Can you work these out from the model? Positions are in its coordinate system, mm. A direction names the side the tool comes from. Give positions to 0.01 mm unless a question says otherwise; leave off trailing zeros. Write each loop counter-clockwise with the first axis right and the second up, starting at its lowest first coordinate (ties: lowest second). Pieces come first, ordered by that corner, then holes.
```python
from build123d import *
from build123d.topology import SkipClean

# Parameters (mm, degrees)
BOSS_EXTRUDE1_DEPTH       = 25.4
F_8_0_18_DIAMETER_HOLE1_D = 4.572
SKETCH8_W                 = 22.225
SKETCH8_H                 = 53.34
CUT_EXTRUDE1_DEPTH        = 74.933200255
CUT_EXTRUDE2_DEPTH        = 74.933200255
FILLET1_R                 = 3.175
FILLET3_R                 = 0.508
FILLET4_R                 = 6.35


with BuildPart() as part:
    # Sketch1 → Boss-Extrude1 (new body)
    with BuildSketch(Plane(origin=(0, 0, 0), x_dir=(0, 0, -1), z_dir=(1, 0, 0))):
        with BuildLine():
            Line((0, 0), (0, 53.34))
            Line((0, 53.34), (-22.225, 53.34))
            Line((-22.225, 53.34), (-22.225, 46.482))
            ThreePointArc((-22.225, 46.482), (-2.413, 26.67), (-22.225, 6.858))
            Line((-22.225, 6.858), (-22.225, 0))
            Line((-22.225, 0), (0, 0))
        make_face()
    boss_extrude1 = extrude(amount=BOSS_EXTRUDE1_DEPTH)

    # #8 (0.18) Diameter Hole1 (through all)
    with Locations(Plane.XY.offset(22.225)):
        with Locations((4.7625, 49.911), (20.6375, 49.911), (20.6375, 3.429), (4.7625, 3.429)):
            f_8_0_18_diameter_hole1 = Hole(F_8_0_18_DIAMETER_HOLE1_D / 2)

    # Mirror1: Boss-Extrude1, #8 (0.18) Diameter Hole1 across plane
    with SkipClean():  # the faces are left unmerged after this step: merging them gives an invalid solid
        add(boss_extrude1.mirror(Plane(origin=(25.4, 53.34, 22.225), x_dir=(1, 0, 0), z_dir=(0, 0, -1))))
        add(f_8_0_18_diameter_hole1.mirror(Plane(origin=(25.4, 53.34, 22.225), x_dir=(1, 0, 0), z_dir=(0, 0, -1))), mode=Mode.SUBTRACT)

    # Sketch8 → Cut-Extrude1 (cut, through all)
    with BuildSketch(Plane.ZY):
        with Locations((11.1125, 26.67)):
            Rectangle(SKETCH8_W, SKETCH8_H)
    extrude(amount=-CUT_EXTRUDE1_DEPTH, mode=Mode.SUBTRACT)

    # Sketch9 → Cut-Extrude2 (cut, through all)
    with BuildSketch(Plane(origin=(25.4, 0, 0), x_dir=(0, 0, -1), z_dir=(1, 0, 0))):
        Polygon((-44.45, 0), (-38.1, 0), (-38.1, 7.62), (-44.45, 25.4), align=None)
    extrude(amount=-CUT_EXTRUDE2_DEPTH, mode=Mode.SUBTRACT)

    # Fillet1
    fillet1_edges = [part.edges().sort_by_distance(p)[0] for p in [
        (0, 0, 30.1625),
        (25.4, 0, 30.1625),
        (0, 53.34, 33.3375),
        (25.4, 53.34, 33.3375),
    ]]
    fillet(fillet1_edges, radius=FILLET1_R)

    # Fillet3
    fillet3_edges = [part.edges().sort_by_distance(p)[0] for p in [
        (0, 37.7825, 44.45),
        (25.4, 37.7825, 44.45),
        (0, 16.51, 41.275),
        (25.4, 16.51, 41.275),
        (12.7, 0, 38.1),
        (12.7, 0, 22.225),
        (25.4, 5.0165, 22.225),
        (0, 5.0165, 22.225),
        (24.47006403, 0.92993597, 22.225),
        (0.92993597, 0.92993597, 22.225),
        (0, 5.3975, 38.1),
        (25.4, 5.3975, 38.1),
        (24.47006403, 0.92993597, 38.1),
        (0.92993597, 0.92993597, 38.1),
        (12.7, 53.34, 44.45),
        (0.92993597, 52.41006403, 44.45),
        (24.47006403, 52.41006403, 44.45),
        (12.7, 53.34, 22.225),
        (0.92993597, 52.41006403, 22.225),
        (24.47006403, 52.41006403, 22.225),
        (25.4, 26.67, 42.037),
        (0, 26.67, 42.037),
        (0, 48.3235, 22.225),
        (12.7, 46.482, 22.225),
        (25.4, 48.3235, 22.225),
        (12.7, 6.858, 22.225),
    ]]
    fillet(fillet3_edges, radius=FILLET3_R)

    # Fillet4
    # the kernel refuses this fillet: 6.35 mm, written as the material it takes off along each edge
    with BuildSketch(Plane(origin=(25.4, 26.499907309, 38.1), x_dir=(0, 0, 1), z_dir=(0, 1, 0))) as fillet4_piece_1:
        with BuildLine():
            CenterArc((5.842, -0.508), 0.508, 0, 90)
            Line((6.35, -0.508), (6.35, 0))
            Line((6.35, 0), (5.842, 0))
        make_face()
    revolve(axis=Axis((25.4, 26.499907309, 38.1), (1, 0, 0)), revolution_arc=19.653824058, mode=Mode.SUBTRACT)
    with BuildSketch(Plane(origin=(0, 26.499907309, 38.1), x_dir=(0, -0.3363363969981563, 0.9417419115948376), z_dir=(0, -0.9417419115948376, -0.3363363969981563))) as fillet4_piece_2:
        with BuildLine():
            CenterArc((5.842, -0.508), 0.508, 0, 90)
            Line((6.35, -0.508), (6.35, 0))
            Line((6.35, 0), (5.842, 0))
        make_face()
    revolve(axis=Axis((0, 26.499907309, 38.1), (-1, 0, 0)), revolution_arc=19.653824058, mode=Mode.SUBTRACT)
    with BuildSketch(Plane(origin=(25.4, 25.4, 44.45), x_dir=(0, 1, 0), z_dir=(-1, 0, 0))) as fillet4_piece_3:
        with BuildLine():
            CenterArc((FILLET4_R * 0.173213749464, FILLET4_R), FILLET4_R, 250.346175942, 19.653824058)
            Line((-FILLET4_R * 0.163122647534, FILLET4_R * 0.0582580884052), (0, 0))
            Line((0, 0), (FILLET4_R * 0.173213749464, 0))
        make_face()
    extrude(amount=25.4, mode=Mode.SUBTRACT)


solid = part.part
```
1) Suppose I cut it at B-B on z = 41. State how many separate pieces and enclosed holes the cut face has, plus the area to 3 significant figures.
Values follow:
separate pieces: 2
enclosed holes: 2
area: 596 mm2
2) If we mould it in two halves opening along Y, with no side actions, what happens to faces 1 (the face through (24.45, 52.43, 33.19)), 2 (the face through (2.582, 4.116, 30.274)), 3 (the face through (12.871, 15.875, 41.048)), 4 (the face through (0, 34, 42))? For each: +Y half, -Y half, draft (parallel to the pull), parting line (faces both ways), or undercut.
Values follow:
face 1: +Y half
face 2: undercut
face 3: -Y half
face 4: draft
3) For pin 1 Ø12 at (x, z) = (3, 34.5) entering from -Y; pin 2 Ø2 at (x, y) = (7, 3) entering from +Z; pin 3 Ø4 at (x, y) = (9, 30) entering from -Z; pin 4 Ø10 at (x, y) = (3.5, 35.5) entering from -Z, each with a flat end and sliding along its axis, tell me the tip position at first contact or that it passes through.
Values follow:
pin 1: stops at y = 0
pin 2: stops at z = 38.1
pin 3: stops at z = 41.31
pin 4: stops at z = 36.41
4) For faces 5 (the face through (13, 50, 22.225)), 6 (the face through (13, 4, 38.1)), which set-ups out of +Z, -Z, +X, -X, +Y, -Y let a thin tool reach every point of the face, with its end or its side?
Values follow:
face 5: -Z, +X, -X, +Y, -Y
face 6: +Z, +X, -X, -Y
5) Suppose I cut it at A-A on x = 19.75. Write out the boundary of the cut face in (y, z) (3 decimals), plus the area to 3 significant figures.
Values follow:
outline: (0, 22.733) arc R0.508 ccw to (0.508, 22.225) - (1.322, 22.225) - (1.322, 38.1) - (0.508, 38.1) arc R0.508 ccw to (0, 37.592) - close; (5.536, 22.225) - (6.356, 22.225) arc R0.508 ccw to (6.864, 22.72) arc R19.812 cw to (46.476, 22.72) arc R0.508 ccw to (46.984, 22.225) - (47.804, 22.225) - (47.804, 44.45) - (26.5, 44.45) arc R6.35 ccw to (24.364, 44.08) - (7.62, 38.1) - (5.536, 38.1) - close; (52.018, 22.225) - (52.832, 22.225) arc R0.508 ccw to (53.34, 22.733) - (53.34, 43.942) arc R0.508 ccw to (52.832, 44.45) - (52.018, 44.45) - close
area: 303 mm2
6) Please list where these lines run through material, in increasing order: L1, parallel to X at y = 50, z = 38; L2, parallel to Y at x = 3, z = 30; L3, parallel to Y at x = 4, z = 27.25.
Values follow:
L1: x = 0 to 2.48, 7.05 to 18.35, 22.92 to 25.4
L2: y = 0 to 1.97, 4.88 to 8.45, 44.89 to 48.46, 51.37 to 53.34
L3: y = 0 to 1.27, 5.58 to 7.51, 45.83 to 47.76, 52.07 to 53.34
